Could you check a few things on this drawing? It's one solid part, dimensions in mm from its lowest x, y, z. A direction names the side the tool comes from. Give positions to 0.01 mm unless a question says otherwise; leave off trailing zeros. Order: outer loops, then holes, each group sorted by start corner. A loop starts at its lowest first (then second) coordinate and runs counter-clockwise, first axis right, second up. Notation, with made-up numbers: (73.5, -7.75) - (106.5, -7.75) arc R6 ccw to (106.5, 0.25) - close; hole circle Ø8 at (69.25, -39). An arc over 180 degrees is marked (long way). Return JSON: item names as keys, results as strings.
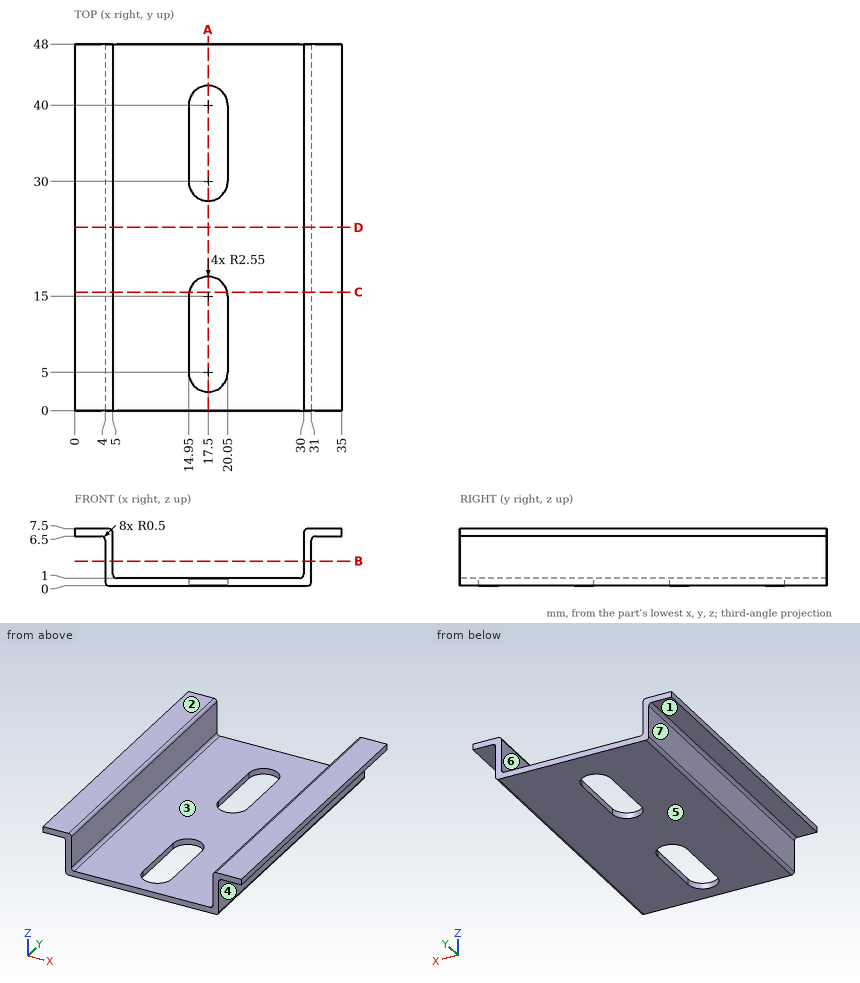
1. For pin 1 Ø1 at (y, z) = (41, 2) entering from -X; pin 2 Ø7 at (x, y) = (21.5, 13.5) entering from +Z; pin 3 Ø3 at (x, y) = (33, 21) entering from -Z, each with a flat end and sliding along its axis, tell me the tip position at first contact or that it passes through.
Checks:
{"pin 1": "x = 4", "pin 2": "z = 1", "pin 3": "z = 6.5"}
2. Suppose I cut it at B-B (z = 3.25). List the corners of the cut face in (x, y) for me, plus the area to 3 significant figures.
Checks:
{"outline": "(4, 0) - (5, 0) - (5, 48) - (4, 48) - close; (30, 0) - (31, 0) - (31, 48) - (30, 48) - close", "area": "96.0 mm^2"}
3. Suppose I cut it at D-D (y = 24). List the corners of the cut face in (x, z) for me.
Checks:
{"outline": "(0, 6.5) - (3.5, 6.5) arc R0.5 cw to (4, 6) - (4, 0.5) arc R0.5 ccw to (4.5, 0) - (30.5, 0) arc R0.5 ccw to (31, 0.5) - (31, 6) arc R0.5 cw to (31.5, 6.5) - (35, 6.5) - (35, 7.5) - (30.5, 7.5) arc R0.5 ccw to (30, 7) - (30, 1.5) arc R0.5 cw to (29.5, 1) - (5.5, 1) arc R0.5 cw to (5, 1.5) - (5, 7) arc R0.5 ccw to (4.5, 7.5) - (0, 7.5) - close"}
4. Suppose I cut it at C-C (y = 15.5). List the corners of the cut face in (x, z) for me.
Checks:
{"outline": "(0, 6.5) - (3.5, 6.5) arc R0.5 cw to (4, 6) - (4, 0.5) arc R0.5 ccw to (4.5, 0) - (15, 0) - (15, 1) - (5.5, 1) arc R0.5 cw to (5, 1.5) - (5, 7) arc R0.5 ccw to (4.5, 7.5) - (0, 7.5) - close; (20, 0) - (30.5, 0) arc R0.5 ccw to (31, 0.5) - (31, 6) arc R0.5 cw to (31.5, 6.5) - (35, 6.5) - (35, 7.5) - (30.5, 7.5) arc R0.5 ccw to (30, 7) - (30, 1.5) arc R0.5 cw to (29.5, 1) - (20, 1) - close"}
5. Thinking about a two-plate mould opening in X: for the marked faces 4, 5, 6 and 7, which applies, +X half, -X half, draft (parallel to the pull), parting line (faces both ways), or undercut?
Checks:
{"face 4": "+X half", "face 5": "draft", "face 6": "undercut", "face 7": "-X half"}
6. On a 3-axis mill with a long thin cutter (end or side, diameter ignored), from which of +Z, -Z, +X, -X, +Y, -Y can I reach the whole of each face in a straight line? I mean the marked faces 1, 2 and 3. Say none if no direction works.
Checks:
{"face 1": "-Z, -X, +Y, -Y", "face 2": "+Z, +X, -X, +Y, -Y", "face 3": "+Z, +Y, -Y"}
7. Suppose I cut it at A-A (x = 17.5). List the corners of the cut face in (y, z) for me.
Checks:
{"outline": "(0, 0) - (2.45, 0) - (2.45, 1) - (0, 1) - close; (17.55, 0) - (27.45, 0) - (27.45, 1) - (17.55, 1) - close; (42.55, 0) - (48, 0) - (48, 1) - (42.55, 1) - close"}
8. If I drill on L1, parallel to X at y = 33, z = 1.75; L2, parallel to Z at x = 11, y = 22.5; L3, parallel to X at y = 37.5, z = 7.25, over which ranges is the centre line in solid material (lowest first)? Write a range as [from, to].
Checks:
{"L1": "[4, 5], [30, 31]", "L2": "[0, 1]", "L3": "[0, 4.93], [30.07, 35]"}
